Could you check a few things on this drawing? It's one solid part, dimensions in mm from its lowest x, y, z. A direction names the side the tool comes from. Give positions to 0.01 mm unless a question says otherwise; leave off trailing zeros. Order: outer loops, then holes, each group sorted by start corner. A loop starts at its lowest first (then second) coordinate and runs counter-clockwise, first axis right, second up. Notation, with made-up numbers: (89, 17) -> (93, 17) arc R21 ccw to (93, 37) -> close; hole circle Ø8 at (28.25, 41). An arc over 180 degrees is marked (long way). Answer as a JSON object with one key per item and string values.
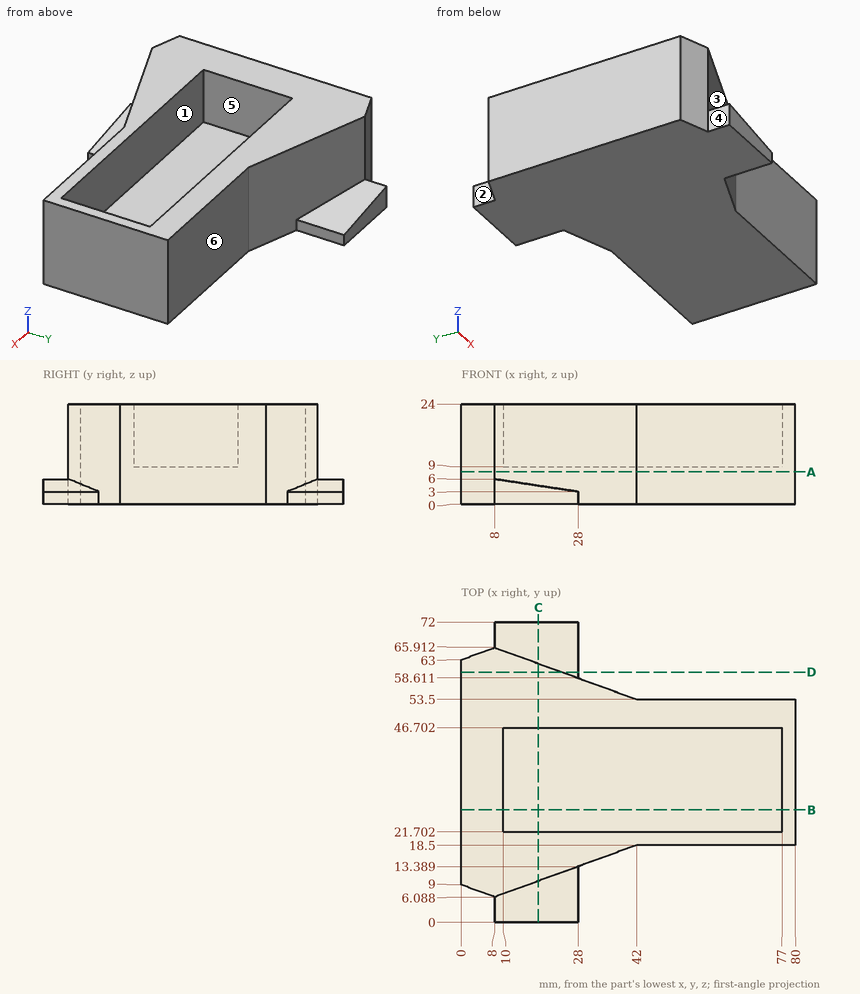
1. If we section it at C-C on x = 18.5: Please give me the cut outline in (y, z) (1 decimal).
Worked answers:
{"outline": "(0, 0) -> (72, 0) -> (72, 4.4) -> (62.1, 4.4) -> (62.1, 24) -> (46.7, 24) -> (46.7, 9) -> (21.7, 9) -> (21.7, 24) -> (9.9, 24) -> (9.9, 4.4) -> (0, 4.4) -> close"}
2. For the marked faces 1, 2 and 3, which set-ups out of +Z, -Z, +X, -X, +Y, -Y let a thin tool reach every point of the face, with its end or its side?
Worked answers:
{"face 1": "+Z", "face 2": "+Z, -Z, -X, +Y", "face 3": "+Z, +X, -Y"}
3. If we section it at A-A on z = 7.75: Please give me the cut outline in (x, y).
Worked answers:
{"outline": "(0, 9) -> (8, 6.09) -> (42, 18.5) -> (80, 18.5) -> (80, 53.5) -> (42, 53.5) -> (8, 65.91) -> (0, 63) -> close"}
4. If we section it at D-D on y = 60: Please give me the cut outline in (x, z), then the cut area to 3 significant figures.
Worked answers:
{"outline": "(0, 0) -> (28, 0) -> (28, 3) -> (24.19, 3.57) -> (24.19, 24) -> (0, 24) -> close", "area": "593 mm²"}
5. If we section it at B-B on y = 27: Please give me the cut outline in (x, z), then the cut area to 3 significant figures.
Worked answers:
{"outline": "(0, 0) -> (80, 0) -> (80, 24) -> (77, 24) -> (77, 9) -> (10, 9) -> (10, 24) -> (0, 24) -> close", "area": "915 mm²"}
6. Will these pins go through, and if not, where does the flat tip stop? pin 1 Ø12 at (x, z) = (66.5, 16) entering from -Y; pin 2 Ø12 at (x, z) = (40.5, 10) entering from +Y; pin 3 Ø20 at (x, y) = (35, 30) entering from +Z; pin 4 Ø2.5 at (y, z) = (68, 1.5) entering from +X.
Worked answers:
{"pin 1": "y = 18.5", "pin 2": "y = 56.24", "pin 3": "z = 24", "pin 4": "x = 28"}
7. Please list where these lines run through material, in increasing order: L1, parallel to Y at x = 56.5, z = 10.5; L2, parallel to Y at x = 72, z = 3.5; L3, parallel to Y at x = 23.5, z = 17.
Worked answers:
{"L1": "18.5 to 21.7, 46.7 to 53.5", "L2": "18.5 to 53.5", "L3": "11.75 to 21.7, 46.7 to 60.25"}
8. If we mould it in two halves opening along Y, with no side actions, what happens to the marked faces 4, 5 and 6? For each: +Y half, -Y half, draft (parallel to the pull), parting line (faces both ways), or undercut.
Worked answers:
{"face 4": "draft", "face 5": "undercut", "face 6": "+Y half"}
